```python
from build123d import *

# Parameters (mm, degrees)
F0_R     = 3.175
F1_DEPTH = 30.48


with BuildPart() as f1:
    # F0 (on Front) → F1 (new body)
    with BuildSketch(Plane.XZ):
        with BuildLine():
            ThreePointArc((3.175, 0), (-2.2450640303, -2.2450640303), (0, 3.175))
            Line((0, 3.175), (0, 9.525))
            ThreePointArc((0, 9.525), (-6.7351920908, 6.7351920908), (-9.525, 0))
            ThreePointArc((-9.525, 0), (-6.7351920908, -6.7351920908), (0, -9.525))
            Line((0, -9.525), (0.6773435479, -9.500885786))
            ThreePointArc((0.6773435479, -9.500885786), (6.9705567315, -6.4912990883), (9.525, 0))
            Line((9.525, 0), (3.175, 0))
        make_face()
        with BuildLine():
            ThreePointArc((-9.525, 0), (-6.7351920908, 6.7351920908), (0, 9.525))
            Line((0, 9.525), (0, 47.625))
            ThreePointArc((0, 47.625), (-10.5003045198, 51.5937314833), (-15.7504812749, 61.51556945))
            Line((-15.7504812749, 61.51556945), (-9.525, 0))
        make_face()
        with BuildLine():
            Line((0, 47.625), (0, 9.525))
            ThreePointArc((0, 9.525), (6.7351920908, 6.7351920908), (9.525, 0))
            Line((9.525, 0), (36.5125, 0))
            ThreePointArc((36.5125, 0), (38.8373399243, 5.6126600757), (44.45, 7.9375))
            Line((44.45, 7.9375), (19.1585847945, 7.9375))
            ThreePointArc((19.1585847945, 7.9375), (13.2627721486, 10.5543077133), (11.2481720528, 16.6820867415))
            Line((11.2481720528, 16.6820867415), (15.7504812749, 61.51556945))
            ThreePointArc((15.7504812749, 61.51556945), (10.5003045198, 51.5937314833), (0, 47.625))
        make_face()
        with BuildLine():
            Line((36.5125, 0), (9.525, 0))
            ThreePointArc((9.525, 0), (6.9705567315, -6.4912990883), (0.6773435479, -9.500885786))
            Line((0.6773435479, -9.500885786), (44.7324052746, -7.9324746146))
            ThreePointArc((44.7324052746, -7.9324746146), (38.9380895153, -5.7116327839), (36.5125, 0))
        make_face()
        with BuildLine():
            ThreePointArc((-15.7504812749, 61.51556945), (-10.5003045198, 51.5937314833), (0, 47.625))
            Line((0, 47.625), (0, 60.325))
            ThreePointArc((0, 60.325), (-3.175, 63.5), (0, 66.675))
            Line((0, 66.675), (0, 79.375))
            ThreePointArc((0, 79.375), (-10.5003045198, 75.4062685167), (-15.7504812749, 65.48443055))
            ThreePointArc((-15.7504812749, 65.48443055), (-15.875, 63.5), (-15.7504812749, 61.51556945))
        make_face()
        with BuildLine():
            Line((0, 60.325), (0, 47.625))
            ThreePointArc((0, 47.625), (10.5003045198, 51.5937314833), (15.7504812749, 61.51556945))
            ThreePointArc((15.7504812749, 61.51556945), (15.8438397373, 62.5058333237), (15.875, 63.5))
            ThreePointArc((15.875, 63.5), (15.8438397373, 64.4941666763), (15.7504812749, 65.48443055))
            ThreePointArc((15.7504812749, 65.48443055), (10.5003045198, 75.4062685167), (0, 79.375))
            Line((0, 79.375), (0, 66.675))
            ThreePointArc((0, 66.675), (2.2450640303, 65.7450640303), (3.175, 63.5))
            ThreePointArc((3.175, 63.5), (2.2450640303, 61.2549359697), (0, 60.325))
        make_face()
        with BuildLine():
            ThreePointArc((44.45, 7.9375), (38.8373399243, 5.6126600757), (36.5125, 0))
            ThreePointArc((36.5125, 0), (38.9380895153, -5.7116327839), (44.7324052746, -7.9324746146))
            ThreePointArc((44.7324052746, -7.9324746146), (50.1616327839, -5.5119104847), (52.3875, 0))
            ThreePointArc((52.3875, 0), (50.0626600757, 5.6126600757), (44.45, 7.9375))
        make_face()
        with BuildLine():
            ThreePointArc((47.625, 0), (44.45, -3.175), (41.275, 0))
            ThreePointArc((41.275, 0), (44.45, 3.175), (47.625, 0))
        make_face(mode=Mode.SUBTRACT)
        with BuildLine():
            ThreePointArc((0, -9.525), (0.3388863295, -9.5189695375), (0.6773435479, -9.500885786))
            Line((0.6773435479, -9.500885786), (0, -9.525))
        make_face()
        with BuildLine():
            Line((-9.4573865922, 115.4329006338), (-15.7504812749, 65.48443055))
            ThreePointArc((-15.7504812749, 65.48443055), (-10.5003045198, 75.4062685167), (0, 79.375))
            Line((0, 79.375), (0, 100.0252))
            Line((0, 100.0252), (0, 104.775))
            ThreePointArc((0, 104.775), (-7.1244825615, 107.9780245784), (-9.4573865922, 115.4329006338))
        make_face()
        with Locations((-3.175, 100.0252)):
            Circle(F0_R, mode=Mode.SUBTRACT)
        with BuildLine():
            Line((0, 100.0252), (0, 79.375))
            ThreePointArc((0, 79.375), (10.5003045198, 75.4062685167), (15.7504812749, 65.48443055))
            Line((15.7504812749, 65.48443055), (9.4573865922, 115.4329006338))
            ThreePointArc((9.4573865922, 115.4329006338), (9.5080816228, 114.8674582405), (9.525, 114.3))
            ThreePointArc((9.525, 114.3), (6.7351920908, 107.5648079092), (0, 104.775))
            Line((0, 104.775), (0, 100.0252))
        make_face()
        with BuildLine():
            ThreePointArc((9.4573865922, 115.4329006338), (0, 123.825), (-9.4573865922, 115.4329006338))
            ThreePointArc((-9.4573865922, 115.4329006338), (-7.1244825615, 107.9780245784), (0, 104.775))
            ThreePointArc((0, 104.775), (6.7351920908, 107.5648079092), (9.525, 114.3))
            ThreePointArc((9.525, 114.3), (9.5080816228, 114.8674582405), (9.4573865922, 115.4329006338))
        make_face()
        with BuildLine():
            ThreePointArc((3.175, 114.3), (2.2450640303, 112.0549359697), (0, 111.125))
            ThreePointArc((0, 111.125), (-2.2450640303, 116.5450640303), (3.175, 114.3))
        make_face(mode=Mode.SUBTRACT)
        with BuildLine():
            Line((0, 9.525), (0, 3.175))
            ThreePointArc((0, 3.175), (2.2450640303, 2.2450640303), (3.175, 0))
            Line((3.175, 0), (9.525, 0))
            ThreePointArc((9.525, 0), (6.7351920908, 6.7351920908), (0, 9.525))
        make_face()
    extrude(amount=F1_DEPTH)


solid = f1.part
```
The listing builds one solid part. Answer for the finished solid, in the listing's coordinates (mm). A direction names the side the tool comes from. Coordinates: 2 decimals unless noted, no trailing zeros. Loops run counter-clockwise (first coordinate to the right, second up) from the corner with the lowest first, then second, coordinate; pieces in that order, holes last. Notation, with made-up numbers: (0, -29) -> (42, -29) arc R13 ccw to (42, -10) -> close; hole circle Ø8 at (-40, 57.25). An arc over 180 degrees is marked (long way). Return JSON: item names as keys, results as strings. Group by question number.
(1) Find the intervals of material crossed by probe 1 along Z at (x, y) = (-2, -21.5); probe 2 along Z at (x, y) = (1, -21.5); probe 3 along X at (y, z) = (-19.5, 114.3) (3 decimals), in increasing order. Write a range as from..to.
(2) A cutting plane is placed at A-A on y = -29. Count the separate pieces of the cut face and the enclosed holes in it, and give its area (3 significant figures).
(3) Which of the six approach directions +Z, -Z, +X, -X, +Y, -Y give full straight-line access (tool end or side, diameter ignored) to faces 5 (the flat face through (32, -15, 7.938)), 6 (the flat face through (13.468, -15.027, 38.785)), 7 (the flat face through (3, -30.48, 43))?
(4) Determine the mould class of faces 1 (the cylindrical face through (0.194, -15.027, 123.823)), 2 (the cylindrical face through (41.52, -15.03, -1.22)), 3 (the cylindrical face through (52.387, -15.027, -0.031)), 4 (the flat face through (3, 0, 43)) for opening direction Z: released by +Z, released by -Z, zero draft, split by the parting line, or undercut.
(5) A cutting plane is placed at B-B on x = 37. Write down the section's boundary in (y, z), and give its area (3 significant figures).
(6) A cutting plane is placed at C-C on z = 48. Write down the section's boundary in (x, y).
(7) Given pin 1 Ø3 at (y, z) = (-21, 69.5) entering from +X; pin 2 Ø4 at (y, z) = (-8, 33.5) entering from -X; pin 3 Ø5 at (x, y) = (39, -7.5) entering from +Z; pin 4 Ø10 at (x, z) = (-3.18, 100.03) entering from +Y, each flat-ended and moving along its own axis, determine where each tip first touches the part or whether it passes through.
The answers:
{
 "1": {"probe 1": "z = -9.31..-2.47, 2.47..61.03, 65.97..97.08, 102.97..111.83, 116.77..123.61", "probe 2": "z = -9.49..-3.01, 3.01..60.49, 66.51..111.29, 117.31..123.77", "probe 3": "x = -9.6..-3.175, 3.175..9.6"},
 "2": {"separate pieces": "1", "enclosed holes": "5", "area": "3,750 mm^2"},
 "3": {"face 5": "+Z, +X, +Y, -Y", "face 6": "+X, +Y, -Y", "face 7": "+Z, -Z, +X, -X, -Y"},
 "4": {"face 1": "released by +Z", "face 2": "undercut", "face 3": "split by the parting line", "face 4": "zero draft"},
 "5": {"outline": "(-30.48, -8.21) -> (0, -8.21) -> (0, 7.94) -> (-30.48, 7.94) -> close", "area": "492 mm^2"},
 "6": {"outline": "(-14.38, -30.48) -> (14.39, -30.48) -> (14.39, 0) -> (-14.38, 0) -> close"},
 "7": {"pin 1": "stops at x = 15.43", "pin 2": "stops at x = -13.12", "pin 3": "stops at z = 7.94", "pin 4": "stops at y = 0"}
}
